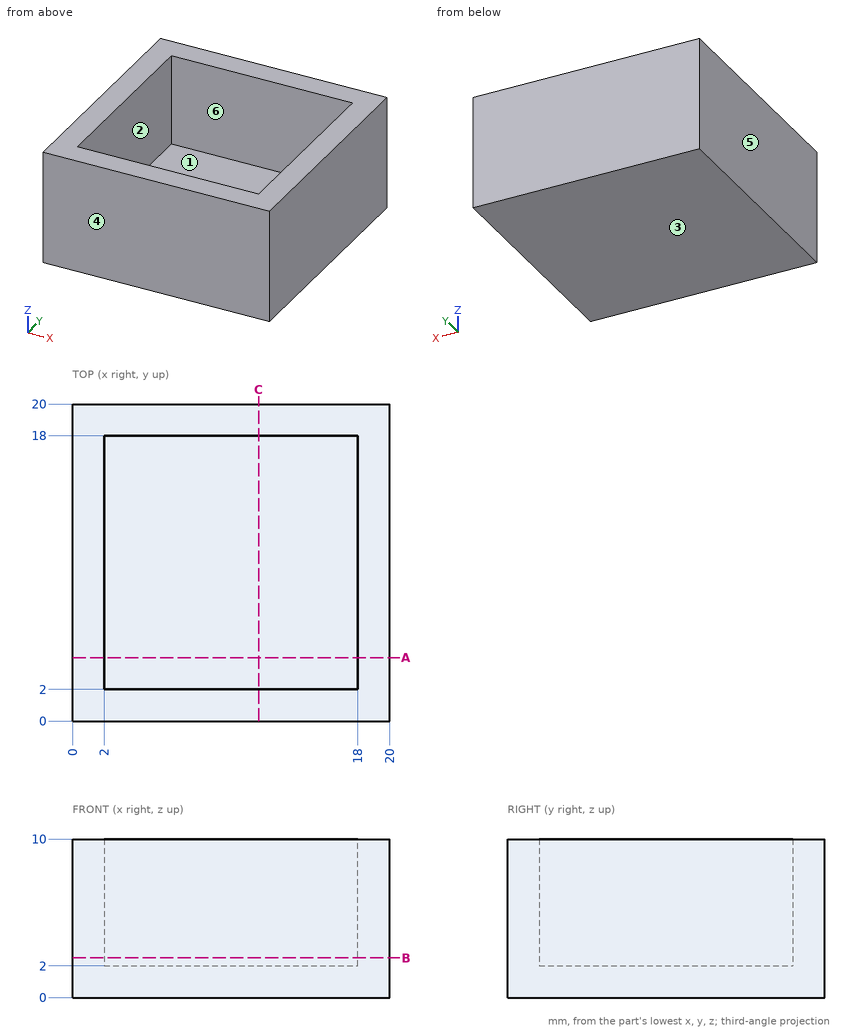
Verification items for this drawing (mm, ordinates from the low corner). A direction names the side the tool comes from. Give positions to 0.01 mm unless a question says otherwise; leave off trailing zeros. Write each loop counter-clockwise with the first axis right and the second up, starting at its lowest first coordinate (ties: lowest second). Pieces come first, ordered by that corner, then holes. Notation, with made-up numbers: (85.25, -21) - (121.25, -21) arc R18 ccw to (121.25, 12) - close; hole circle Ø6 at (-39, -12.5). An arc over 180 degrees is marked (long way). Answer as a JSON object with one key per item and string values. Group by question number.
1) Access from +Z, -Z, +X, -X, +Y, -Y to the whole of each face (thin tool, end or side, straight path). Record for the marked faces 5 and 6.
2) Sectioned sample at B-B (z = 2.5). Record the cut outline in (x, y), then the cut area to 3 significant figures.
3) Thickness scan on probe 1 along X at (y, z) = (7.75, 5.75); probe 2 along Z at (x, y) = (8, 7.5). Record the ranges inside material, lowest first. Write a range as from..to.
4) Release check for a two-part mould opening along Y. For the marked faces 1, 2, 3 and 4 record: pulls with the +Y half, pulls with the -Y half, needs draft (parallel to the pull), parting line crosses it, or undercut.
5) Sectioned sample at A-A (y = 4). Record the cut outline in (x, z).
6) Depth check by flat-ended pin: P1, Ø5, axis at x = 13.5, y = 5, coming from the +Z side. Enter the tip coordinate at first touch or a pass-through.
Geometry results:
{
 "1": {"face 5": "+Z, -Z, -X, +Y, -Y", "face 6": "+Z"},
 "2": {"outline": "(0, 0) - (20, 0) - (20, 20) - (0, 20) - close; hole (2, 2) - (18, 2) - (18, 18) - (2, 18) - close", "area": "144 mm^2"},
 "3": {"probe 1": "x = 0..2, 18..20", "probe 2": "z = 0..2"},
 "4": {"face 1": "undercut", "face 2": "undercut", "face 3": "needs draft", "face 4": "pulls with the -Y half"},
 "5": {"outline": "(0, 0) - (20, 0) - (20, 10) - (18, 10) - (18, 2) - (2, 2) - (2, 10) - (0, 10) - close"},
 "6": {"P1": "stops at z = 2"}
}
